Read the model definition and answer for the solid it produces. Units are mm, in the model's axes. A direction names the side the tool comes from. Round coordinates to 2 decimals unless told otherwise and drop trailing zeros. Write each loop counter-clockwise with the first axis right and the second up, starting at its lowest first coordinate (ties: lowest second). Pieces come first, ordered by that corner, then holes. Notation, with made-up numbers: M 44,4.5 L 48,4.5 A20 cw 48,43.5 Z; hole C 81,-23 d11. An arc over 180 degrees is marked long. Use one line per item in the form item = value. Start each with the question number.
```python
from build123d import *

# Parameters (mm, degrees)
SKETCH1_R                                      = 10
SKETCH1_R_2                                    = 3
SKETCH1_R_3                                    = 1.6
BOSS_EXTRUDE1_DEPTH                            = 10
SKETCH2_R                                      = 5
CUT_EXTRUDE1_DEPTH                             = 6
CSK_FOR_M3_FLAT_HEAD_MACHINE_SCREW1_AT_2_COUNT = 2
CSK_FOR_M3_FLAT_HEAD_MACHINE_SCREW1_AT_2_PITCH = 20


with BuildPart() as part:
    # Sketch1 → Boss-Extrude1 (new body)
    with BuildSketch(Plane(origin=(0, 0, 0), x_dir=(1, 0, 0), z_dir=(0, 1, 0))):
        with Locations((-30, 0)):
            Circle(SKETCH1_R)
        with Locations((-30, 0)):
            Circle(SKETCH1_R_2, mode=Mode.SUBTRACT)
        with BuildLine():
            Line((29.999999936, 10), (-30, 10))
            ThreePointArc((-30, 10), (-22.928932188, 7.071067812), (-20, 0))
            ThreePointArc((-20, 0), (-22.928932188, -7.071067812), (-30, -10))
            Line((-30, -10), (30, -10))
            ThreePointArc((30, -10), (20, -3.2e-08), (29.999999936, 10))
        make_face()
        with Locations((-10, 0)):
            Circle(SKETCH1_R_3, mode=Mode.SUBTRACT)
        with Locations((10, 0)):
            Circle(SKETCH1_R_3, mode=Mode.SUBTRACT)
        with Locations((30, 0)):
            Circle(SKETCH1_R)
        with Locations((30, 0)):
            Circle(SKETCH1_R_2, mode=Mode.SUBTRACT)
    extrude(amount=BOSS_EXTRUDE1_DEPTH)

    # Sketch2 → Cut-Extrude1 (cut)
    with BuildSketch(Plane(origin=(0, 10, 0), x_dir=(1, 0, 0), z_dir=(0, 1, 0))):
        with Locations((-30, 0)):
            Circle(SKETCH2_R)
        with Locations((30, 0)):
            Circle(SKETCH2_R)
    extrude(amount=-CUT_EXTRUDE1_DEPTH, mode=Mode.SUBTRACT)

    # Sketch4 → CSK for M3 Flat Head Machine Screw1 (revolve, cut)
    with BuildSketch(Plane(origin=(-10, 0, 0), x_dir=(0, 0, -1), z_dir=(1, 0, 0))):
        Polygon((0, 0), (0, 10), (1.5, 10), (1.5, 1.8), (3, 0.3), (3, 0), align=None)
    csk_for_m3_flat_head_machine_screw1 = revolve(axis=Axis((-10, -6.35, 0), (0, 1, 0)), mode=Mode.SUBTRACT)

    # CSK for M3 Flat Head Machine Screw1 at 2: CSK for M3 Flat Head Machine Screw1 ×2
    with Locations(*[(i * CSK_FOR_M3_FLAT_HEAD_MACHINE_SCREW1_AT_2_PITCH, 0, 0) for i in range(1, CSK_FOR_M3_FLAT_HEAD_MACHINE_SCREW1_AT_2_COUNT)]):
        add(csk_for_m3_flat_head_machine_screw1, mode=Mode.SUBTRACT)


solid = part.part
```
Q1. Find section D-D on x = -28.5. Write down the section's boundary in (y, z).
Q2. Find section A-A on x = -10. Write down the section's boundary in (y, z), and give its area (3 significant figures).
Q3. Each of these flat-tipped pins is pushed along its axis until it touches: pin 1 Ø5.5 at (x, z) = (30, 0) entering from -Y; pin 2 Ø1.5 at (y, z) = (4, 7) entering from +X; pin 3 Ø4 at (x, z) = (10, 0) entering from -Y; pin 4 Ø9.5 at (x, z) = (-30, 0) entering from +Y. Where does it stop, or does it pass through?
Q4. Straight lines are drawn through the part: line 1 (X direction, y = 0.15, z = 0); line 2 (X direction, y = 7.75, z = 0); line 3 (Z direction, x = -30, y = 5.2). For each, find the intervals that lie inside material, in ascending order. Write a range as [from, to].
Q5. A tool of negligible diameter and unlimited length cuts with its end or side. For faces 1 (the face through (27, 2, 0)), 2 (the face through (7.47, 0.15, -1.61)), 3 (the face through (29.9, 4, 3.3)), from which of +Z, -Z, +X, -X, +Y, -Y can it reach the whole face along a straight path? Write none if from no direction.
Q6. For a pull along X with two mould halves and no side action, classify faces 4 (the face through (-40, 5, 0)), 5 (the face through (-11.6, 5.79, -0.07)), 6 (the face through (-33, 2, 0)), 7 (the face through (0, 5, 10)) as +X half, -X half, draft (parallel to the pull), parting line (faces both ways), or undercut.
Q7. Find section B-B on y = 2.5. Write down the section's boundary in (x, z), and give its area (3 significant figures).
Q8. Find section C-C on z = 0. Count the separate pieces of the cut face and the enclosed holes in it, and give its area (3 significant figures).
Response:
q1.outline = M 0,-10 L 10,-10 L 10,-4.77 L 4,-4.77 L 4,-2.6 L 0,-2.6 Z; M 0,2.6 L 4,2.6 L 4,4.77 L 10,4.77 L 10,10 L 0,10 Z
q2.outline = M 0,-10 L 10,-10 L 10,-1.6 L 1.7,-1.6 L 0.3,-3 L 0,-3 Z; M 0,3 L 0.3,3 L 1.7,1.6 L 10,1.6 L 10,10 L 0,10 Z
q2.area = 165 mm²
q3.pin_1 = through
q3.pin_2 = 37.81
q3.pin_3 = 1.3
q3.pin_4 = 4
q4.line_1 = [-40, -33], [-27, -13], [-7, 7], [13, 27], [33, 40]
q4.line_2 = [-40, -35], [-25, -11.6], [-8.4, 8.4], [11.6, 25], [35, 40]
q4.line_3 = [-10, -5], [5, 10]
q5.face_1 = +Y, -Y
q5.face_2 = -Y
q5.face_3 = +Y
q6.face_4 = -X half
q6.face_5 = undercut
q6.face_6 = undercut
q6.face_7 = draft
q7.outline = M -30,-10 L 30,-10 A10 ccw 30,10 L -30,10 A10 ccw Z; hole C -30,0 d6; hole C -10,0 d3.2; hole C 10,0 d3.2; hole C 30,0 d6
q7.area = 1,440 mm²
q8.separate_pieces = 5
q8.enclosed_holes = 0
q8.area = 562 mm²
